For this review, use the dimensioned drawing (mm, ordinates from the lowest corner) and the shaded views. Coordinates: 2 decimals unless noted, no trailing zeros. Write each loop counter-clockwise with the first axis right and the second up, starting at its lowest first coordinate (ties: lowest second). Pieces come first, ordered by that corner, then holes.
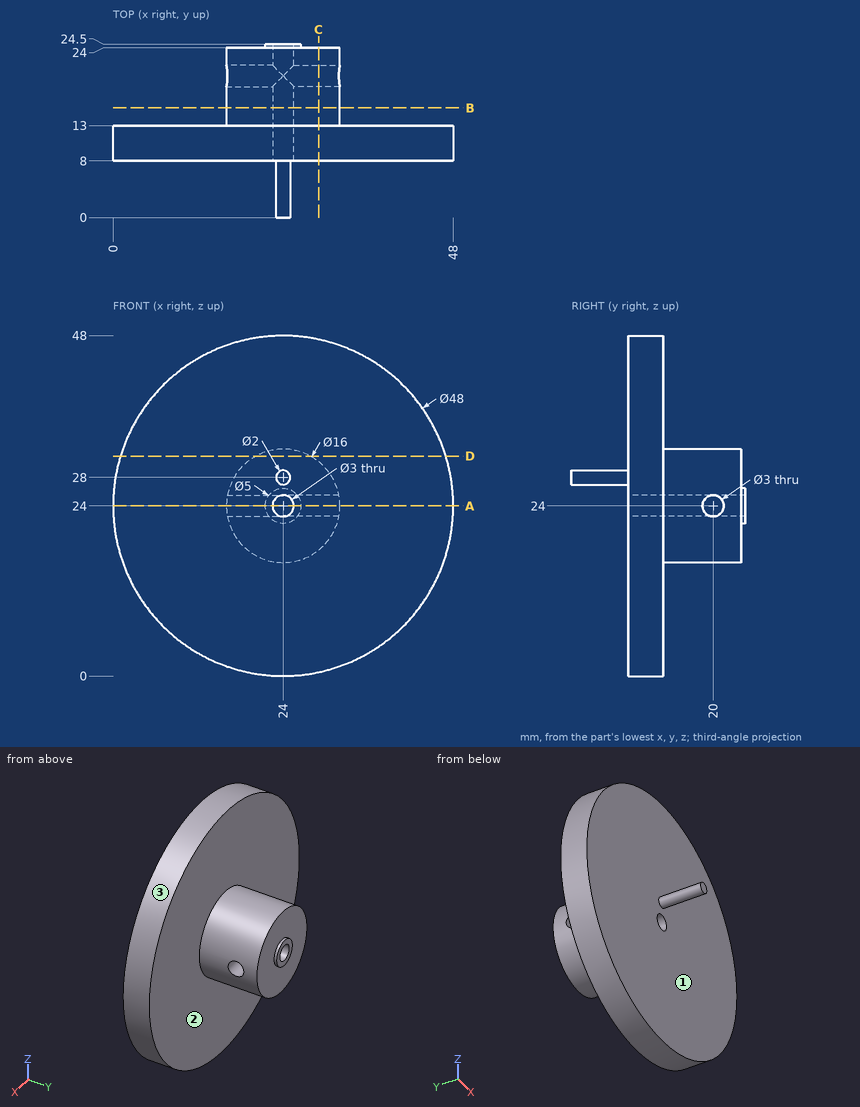
Item 1: Take a section at A-A, the plane z = 24. Write out the cut boundary in (x, y), plus the area to 3 significant figures.
Solved:
outline: (0, 8) - (22.5, 8) - (22.5, 18.5) - (16, 18.5) - (16, 13) - (0, 13) - close; (16, 21.5) - (22.5, 21.5) - (22.5, 24.5) - (21.5, 24.5) - (21.5, 24) - (16, 24) - close; (25.5, 8) - (48, 8) - (48, 13) - (32, 13) - (32, 18.5) - (25.5, 18.5) - close; (25.5, 21.5) - (32, 21.5) - (32, 24) - (26.5, 24) - (26.5, 24.5) - (25.5, 24.5) - close
area: 330 mm2
Item 2: For pin 1 (5 mm diameter, centred on y = 20, z = 24, fed in from -X); pin 2 (12 mm diameter, centred on x = 40.5, z = 33.5, fed in from -Y); pin 3 (8 mm diameter, centred on y = 11.5, z = 34.5, fed in from -X), all flat-tipped, find the tip position at first contact; note any pin that passes through.
Solved:
pin 1: stops at x = 16
pin 2: stops at y = 8
pin 3: stops at x = 0.9
Item 3: Take a section at D-D, the plane z = 31. Write out the cut boundary in (x, y).
Solved:
outline: (1.04, 8) - (46.96, 8) - (46.96, 13) - (27.87, 13) - (27.87, 24) - (20.13, 24) - (20.13, 13) - (1.04, 13) - close
Item 4: Take a section at C-C, the plane x = 29. Write out the cut boundary in (y, z) (3 decimals).
Solved:
outline: (8, 0.527) - (13, 0.527) - (13, 17.755) - (24, 17.755) - (24, 30.245) - (13, 30.245) - (13, 47.473) - (8, 47.473) - close; hole circle Ø3 at (20, 24)
Item 5: To check wall thickness, follow line 1 along Z through (x, y) = (24, 22.1); line 2 along Y through (x, z) = (4.5, 15). State the ranges of each line that lie inside material, in increasing order.
Solved:
line 1: z = 16 to 22.5, 25.5 to 32
line 2: y = 8 to 13
Item 6: Take a section at B-B, the plane y = 15.5. Write out the cut boundary in (x, z).
Solved:
outline: circle Ø16 at (24, 24); hole circle Ø3 at (24, 24)
Item 7: Mouldability with a two-part tool opening along Y and no side actions: class the marked faces 1, 2 and 3 as pulls with the +Y half, pulls with the -Y half, needs draft (parallel to the pull), parting line crosses it, or undercut.
Solved:
face 1: pulls with the -Y half
face 2: pulls with the +Y half
face 3: needs draft
